from build123d import *

# Parameters (mm, degrees)
F2_DEPTH  = 1.524
F3_W      = 519.1125
F3_H      = 25.4
F4_DEPTH  = 1.524
F6_DEPTH  = 50.8
F8_DEPTH  = 685.801
F10_DEPTH = 304.801


# Not quite as in the source:
# - a variable given as a bare number and used for a length is read in inches; the dataset says mm whatever the document's units were


with BuildPart() as f2:
    # F1 (on Top) → F2 (new body)
    with BuildSketch(Plane.XY):
        Polygon((0, 0), (-152.4021759864, 0), (-298.4521759864, -146.05), (-304.8, -146.2162236218), (-291.2112189215, -665.1508367331), (-284.8633949079, -664.9846131114), (-284.3183248194, -685.8), (0, -685.8), align=None)
    extrude(amount=F2_DEPTH)

    # F3 (on face) → F4 (join)
    with BuildSketch(Plane(origin=(-308.4173240373, -8.0761918578, 0), x_dir=(0.0261769483, -0.999657325, 0), z_dir=(-0.999657325, -0.0261769483, 0))):
        with Locations((397.7436351295, -11.176)):
            Rectangle(F3_W, F3_H)
    extrude(amount=-F4_DEPTH)

    # F5 (on Top) → F6 (join)
    with BuildSketch(Plane.XY):
        Polygon((-152.4021759864, 0), (-298.4521759864, -146.05), (-297.3745452519, -147.1276307345), (-151.3245452519, -1.0776307345), align=None)
    extrude(amount=F6_DEPTH)

    # F7 (on Front) → F8 (cut, through all)
    with BuildSketch(Plane.XZ):
        Polygon((6.35, 4.6485226281), (-17.3485226281, 4.6485226281), (6.35, -1.7014773719), align=None)
    extrude(amount=F8_DEPTH, mode=Mode.SUBTRACT)

    # F9 (on Right) → F10 (cut, through all)
    with BuildSketch(Plane.YZ):
        Polygon((-668.4514773719, 4.6485226281), (-692.15, 4.6485226281), (-692.15, -1.7014773719), align=None)
    extrude(amount=-F10_DEPTH, mode=Mode.SUBTRACT)


solid = f2.part
Here's how the part is built. I have some questions about the finished solid (model axes, mm). A direction names the side the tool comes from. Coordinates: 2 decimals unless noted, no trailing zeros. Loops run counter-clockwise (first coordinate to the right, second up) from the corner with the lowest first, then second, coordinate; pieces in that order, holes last.
1. For P1, Ø1.5, axis at x = -179.5, y = -177, coming from the +Z side; P2, Ø1.5, axis at x = -65.5, y = -413.5, coming from the -Z side; P3, Ø1, axis at y = -357, z = -6, coming from the -X side, each with a flat end and sliding along its axis, tell me the tip position at first contact or that it passes through.
2. I need wall thicknesses on L1, parallel to Z at x = -202, y = -513.5; L2, parallel to Y at x = -226, z = 10; L3, parallel to X at y = -50.5, z = 37. Which ranges of each line are inside material? Lowest first, please.
3. Imagine slicing it at B-B, the plane x = -137.5. Please give me the cut outline in (y, z).
4. Imagine slicing it at C-C, the plane z = 22. Please give me the cut outline in (x, y).
5. For faces 1 (the flat face through (-224.4, -72, 25)), 2 (the flat face through (-157, -335, 1.524)), which set-ups out of +Z, -Z, +X, -X, +Y, -Y let a thin tool reach every point of the face, with its end or its side?
6. Imagine slicing it at A-A, the plane y = -360. Please give me the cut outline in (x, z), and give its area (3 significant figures).
7. Imagine slicing it at D-D, the plane x = -259. Please give me the cut outline in (y, z).
Taken from the geometry:
1. P1: stops at z = 1.52
1. P2: stops at z = 0
1. P3: stops at x = -299.29
2. L1: z = 0 to 1.52
2. L2: y = -75.75 to -73.6
2. L3: x = -202.9 to -200.75
3. outline: (-685.8, 0) - (0, 0) - (0, 1.52) - (-680.11, 1.52) - close
4. outline: (-298.45, -146.05) - (-297.37, -147.13) - (-151.32, -1.08) - (-152.4, 0) - close
5. face 1: +Z, -Z, -X, +Y
5. face 2: +Z, +X, -Y
6. outline: (-299.2, -23.88) - (-297.68, -23.88) - (-297.68, 0) - (0, 0) - (-5.69, 1.52) - (-299.2, 1.52) - close
6. area: 488 mm2
7. outline: (-685.8, 0) - (-106.6, 0) - (-106.6, 50.8) - (-108.75, 50.8) - (-108.75, 1.52) - (-680.11, 1.52) - close
